Design review of the part shown in the three views and the two pictorial views. Dimensions are in mm from the part's minimum x, y and z. A direction names the side the tool comes from. Round coordinates to 2 decimals unless told otherwise and drop trailing zeros. Write each loop counter-clockwise with the first axis right and the second up, starting at its lowest first coordinate (ties: lowest second). Pieces come first, ordered by that corner, then holes. Notation, with made-up numbers: (-31.5, -14.5) -> (2.5, -14.5) arc R26 ccw to (2.5, 8.5) -> close; hole circle Ø7 at (0, -34). An arc over 180 degrees is marked (long way). Return JSON: item names as keys, results as strings. Group by question number.
1. Tool access review of the marked faces 4 and 5: name each direction out of +Z, -Z, +X, -X, +Y, -Y from which nothing blocks a thin tool from reaching the whole face with its end or side.
2. Take a section at B-B, the plane z = 8. Write out the cut boundary in (x, y).
3. For line 1 along X through (y, z) = (6, 8); line 2 along Y through (x, z) = (14, 9.75), list the stretches that pass through material, from the lowest coordinate up. Write a range as from..to.
4. Take a section at C-C, the plane y = 10. Write out the cut boundary in (x, z), then the cut area to 3 significant figures.
5. Mouldability with a two-part tool opening along Y and no side actions: class the marked faces 1, 2 and 3 as pulls with the +Y half, pulls with the -Y half, needs draft (parallel to the pull), parting line crosses it, or undercut.
6. Clearance check with flat-ended pins moving along their axes: P1, Ø5, axis at x = 10, z = 5.5, coming from the +Y side; P2, Ø1.5, axis at y = 12, z = 3.5, coming from the +X side; P3, Ø1, axis at y = 1.5, z = 3.5, coming from the +X side; P4, Ø2, axis at x = 10, y = 6.5, coming from the +Z side. State where each tip first meets the part, or that it passes through.
7. Take a section at A-A, the plane x = 8. Write out the cut boundary in (y, z).
8. Take a section at D-D, the plane y = 12.25. Write out the cut boundary in (x, z).
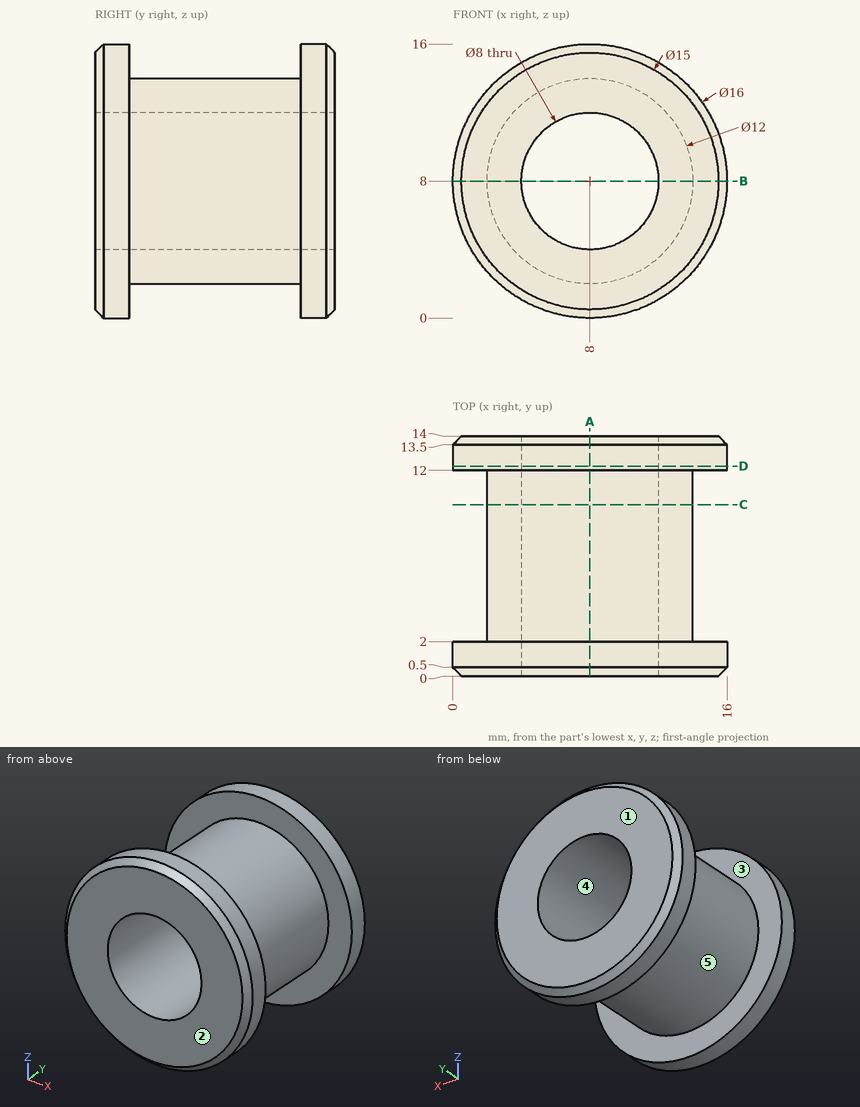
Output:
{
 "1": {"face 4": "+Y, -Y", "face 5": "none"},
 "2": {"outline": "(0, 0.5) -> (0.5, 0) -> (4, 0) -> (4, 14) -> (0.5, 14) -> (0, 13.5) -> (0, 12) -> (2, 12) -> (2, 2) -> (0, 2) -> close; (12, 0) -> (15.5, 0) -> (16, 0.5) -> (16, 2) -> (14, 2) -> (14, 12) -> (16, 12) -> (16, 13.5) -> (15.5, 14) -> (12, 14) -> close"},
 "3": {"line 1": "x = 2..4, 12..14", "line 2": "y = 0..2, 12..14"},
 "4": {"outline": "circle Ø12 at (8, 8); hole circle Ø8 at (8, 8)", "area": "62.8 mm^2"},
 "5": {"face 1": "pulls with the +Y half", "face 2": "pulls with the -Y half", "face 3": "undercut"},
 "6": {"P1": "stops at y = 14", "P2": "stops at x = 15.07", "P3": "stops at x = 14.93", "P4": "stops at z = 13.92"},
 "7": {"outline": "(0, 0.5) -> (0.5, 0) -> (2, 0) -> (2, 2) -> (12, 2) -> (12, 0) -> (13.5, 0) -> (14, 0.5) -> (14, 4) -> (0, 4) -> close; (0, 12) -> (14, 12) -> (14, 15.5) -> (13.5, 16) -> (12, 16) -> (12, 14) -> (2, 14) -> (2, 16) -> (0.5, 16) -> (0, 15.5) -> close"},
 "8": {"outline": "circle Ø16 at (8, 8); hole circle Ø8 at (8, 8)"}
}
